Autodesk Inventor part; units mm, degrees
ref_plane "Startebene" through (0, 0, 0) normal (0, 0, 1) x (1, 0, 0)
ref_plane "Endebene" through (0, 0, 70) normal (0, 0, 1) x (1, 0, 0)
ref_plane "YZ Plane" through (0, 0, 0) normal (1, 0, 0) x (0, 1, 0)
ref_plane "Startebene" through (0, 0, 0) normal (0, 0, 1) x (1, 0, 0)
ref_plane "Endebene" through (0, 0, 70) normal (0, 0, 1) x (1, 0, 0)
sketch "Skizze" plane through (0, 0, 0) normal (0, 0, 1) x (1, 0, 0)
  line L0 (4, -20) -> (-4, -20)
  line L1 (-4, -20) -> (-4, 20)
  line L2 (-4, 20) -> (4, 20)
  line L3 (4, 20) -> (4, -20)
  line L4 (-6, 0) -> (8, 0) construction
  line L5 (0, -30) -> (0, 40) construction
  line L6 (0, 54) -> (0, -44) construction
  line L7 (-9.2, 0) -> (13.2, 0) construction
  dimension "d0" = 40
  dimension "d1" = 8
  dimension "d4" = 4
  dimension "d5" = 20
extrude "Körper" add sketch "Skizze" along normal up to surface (70 mm away) from surface at 0
sketch "Sketch3" plane through (0, 0, 0) normal (0, 0, 1) x (1, 0, 0)
  line L0 (0, 0) -> (10, 0)
ref_plane "Work Plane3" through (0, 0, 0) normal (0, -1, 0) x (1, 0, 0)
sketch "Sketch4" plane through (0, 0, 0) normal (0, -1, 0) x (1, 0, 0)
  line L0 (-2, 0) -> (12, 0)
  line L1 (-2, 70) -> (12, 70)
  dimension "d9" = 70
sketch "Skizze5" plane through (4, -20, 70) normal (1, 0, 0) x (0, 0, -1)
  line L0 (70, 0) -> (0, 0)
  line L1 (70, 40) -> (70, 0)
  point P0 (70, 20)
  point P1 (50, 20)
  dimension "d11" = 20
  dimension "d19" = 20
hole "Bohrung1" at (4, 0, 20) direction (-1, 0, 0) diameter 16 depth 15 tip angle 118
sketch "Skizze6" plane through (4, -20, 70) normal (1, 0, 0) x (0, 0, -1)
  circle A0 centre (50, 20) radius 8
  line L0 (70, 40) -> (0, 40)
  line L1 (70, 0) -> (30, 0)
  line L2 (30, 0) -> (30, 40)
  line L3 (30, 40) -> (70, 40)
  line L4 (70, 40) -> (70, 0)
  point P0 (70, 20)
  dimension "d20" = 40
extrude "Extrusion2" cut sketch "Skizze6" against normal blind 1
sketch "Skizze7" plane through (-4, 20, 0) normal (-1, 0, 0) x (0, 0, 1)
  circle A0 centre (20, -20) radius 8
  line L0 (0, -40) -> (70, -40)
  line L1 (0, 0) -> (40, 0)
  line L2 (40, 0) -> (40, -40)
  line L3 (40, -40) -> (0, -40)
  line L4 (0, -40) -> (0, 0)
  point P0 (0, -20)
  dimension "d23" = 40
extrude "Extrusion3" cut sketch "Skizze7" against normal blind 1
equation "\"d0\" = G_W"
equation "\"d1\" = G_H"
equation "\"d4\" = 0.5 * d1"
equation "\"d5\" = 0.5 * d0"
equation "\"d2\" = G_L"
equation "\"G_W\" = 40"
equation "\"G_H\" = 8"
equation "\"G_L\" = d9"
equation "\"G_OFFSET_START\" = 0"
equation "\"G_OFFSET_END\" = 0"
properties part number "EN 10058 - 40 x 6 - 60" material "Stahl, weich"
Design review of the part built by this model. Coordinates are the model's own, in mm. A direction names the side the tool comes from. Coordinates: 2 decimals unless noted, no trailing zeros. Order: outer loops, then holes, each group sorted by start corner. A loop starts at its lowest first (then second) coordinate and runs counter-clockwise, first axis right, second up. Notation, with made-up numbers: (-33, 18.5) - (-10, 18.5) arc R16 ccw to (-10, 39.5) - close; hole circle Ø11 at (37, 62.5). An arc over 180 degrees is marked (long way). Answer in a Markdown table with one row per item.
(1) Consider section B-B on y = 0. State the section outline as (x, z) points.
Checked values:
| item | result |
|---|---|
| outline | (-4, 40) - (-3, 40) - (-3, 28) - (3, 28) - (3, 40) - (4, 40) - (4, 70) - (-4, 70) - close; (-3, 0) - (3, 0) - (3, 12) - (-3, 12) - close |
(2) For faces 4 (the flat face through (3, 0, 11)), 5 (the flat face through (0, -20, 35)), 6 (the flat face through (-3, 0, 29)), list the 3-axis set-ups (+Z, -Z, +X, -X, +Y, -Y) from which the entire face can be reached by the end or side of a thin tool; tool diameter is ignored.
Checked values:
| item | result |
|---|---|
| face 4 | -Z, +X, +Y, -Y |
| face 5 | +Z, -Z, +X, -X, -Y |
| face 6 | -Z, -X, +Y, -Y |
(3) Consider section A-A on z = 20. State the section outline as (x, y) points.
Checked values:
| item | result |
|---|---|
| outline | (-3, -20) - (3, -20) - (3, -8) - (-3, -8) - close; (-3, 8) - (3, 8) - (3, 20) - (-3, 20) - close |
(4) Clearance check with flat-ended pins moving along their axes: pin 1 (2 mm diameter, centred on y = -11, z = 35, fed in from +X); pin 2 (0.5 mm diameter, centred on x = -3.5, y = 4, fed in from -Z); pin 3 (4 mm diameter, centred on x = 0, y = -10, fed in from -Z); pin 4 (9.5 mm diameter, centred on y = 0, z = 20, fed in from +X). State where each tip first meets the part, or that it passes through.
Checked values:
| item | result |
|---|---|
| pin 1 | x = 3 |
| pin 2 | z = 40 |
| pin 3 | z = 0 |
| pin 4 | through |
(5) The part is to be moulded in two halves that separate along Z. For faces 1 (the cylindrical face through (-0.042, 4.868, 26.349)), 2 (the flat face through (4, 0, 55)), 3 (the flat face through (0, 0, 0)), say which applies: released by +Z, released by -Z, zero draft, split by the parting line, or undercut.
Checked values:
| item | result |
|---|---|
| face 1 | undercut |
| face 2 | zero draft |
| face 3 | released by -Z |
(6) Consider section C-C on x = 2.25. State the section outline as (y, z) points, plus the area to 3 significant figures.
Checked values:
| item | result |
|---|---|
| outline | (-20, 0) - (20, 0) - (20, 70) - (-20, 70) - close; hole circle Ø16 at (0, 20) |
| area | 2,600 mm^2 |
(7) Consider section D-D on z = 35.5. State the section outline as (x, y) points.
Checked values:
| item | result |
|---|---|
| outline | (-3, -20) - (3, -20) - (3, 20) - (-3, 20) - close |
(8) Wall thickness on line 1 along Y through (x, z) = (0.9, 20); line 2 along X through (y, z) = (18.5, 14.5); line 3 along Z through (x, y) = (2.25, 3): over which ranges is each line inside the solid? List them lowest first. Write a range as from..to.
Checked values:
| item | result |
|---|---|
| line 1 | -20..-8, 8..20 |
| line 2 | -3..3 |
| line 3 | 0..12.58, 27.42..70 |
